Read the model definition and answer for the solid it produces. Units are mm, in the model's axes. Coordinates: 2 decimals unless noted, no trailing zeros. Order: outer loops, then holes, each group sorted by start corner. A loop starts at its lowest first (then second) coordinate and runs counter-clockwise, first axis right, second up.
Autodesk Inventor part; units mm, degrees
ref_plane "YZ Plane" through (0, 0, 0) normal (1, 0, 0) x (0, 1, 0)
ref_plane "XZ Plane" through (0, 0, 0) normal (0, 1, 0) x (-1, 0, 0)
ref_plane "XY Plane" through (0, 0, 0) normal (0, 0, 1) x (1, 0, 0)
sketch "Sketch1" plane through (0, 0, 0) normal (1, 0, 0) x (0, 1, 0)
  line L0 (-8.4509, -132.8176) -> (-8.4509, 317.1824)
  line L1 (-8.4509, 317.1824) -> (49.5047, 301.6533)
  line L2 (-8.4509, 317.1824) -> (51.5491, 317.1824) construction
  line L3 (49.5047, 301.6533) -> (49.5047, -128.3467)
  line L4 (49.5047, -128.3467) -> (-8.4509, -132.8176)
  point P0 (0, 0)
  dimension "d0" = 450
  dimension "d1" = 60
  dimension "d2" = 15
  dimension "d3" = 430
extrude "Extrusion1" add sketch "Sketch1" along normal blind 300
fillet "Fillet1" radius 5 2 edges at (150, -8.4509, 317.1824) (150, -8.4509, -132.8176)
fillet "Fillet2" radius 10 2 edges at (150, 49.5047, 301.6533) (150, 49.5047, -128.3467)
properties part number "Chassisew" material "Iron, Gray"
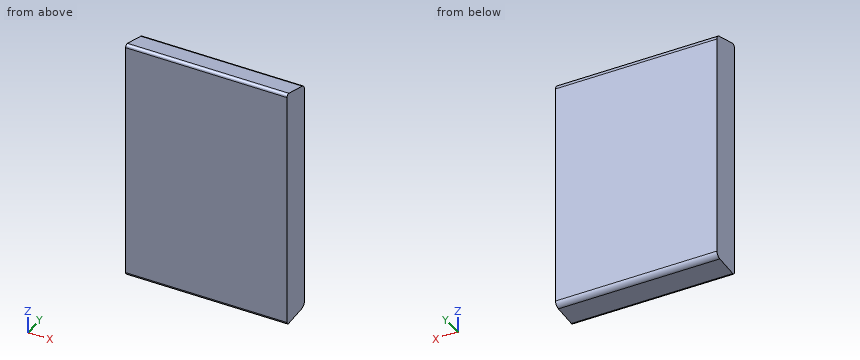
1) Straight lines are drawn through the part: line 1 (Z direction, x = 140.5, y = 21.5); line 2 (Z direction, x = 200, y = 26.5). For each, find the intervals that lie inside material, in ascending order.
A:
line 1: z = -130.51 to 309.16
line 2: z = -130.12 to 307.82
2) A cutting plane is placed at B-B, the plane y = 31. Determine the outline of the cut face in (x, z), and give its area (3 significant figures).
A:
outline: (0, -129.77) - (300, -129.77) - (300, 306.61) - (0, 306.61) - close
area: 131,000 mm2
3) Flat-ended cylindrical pins translate along their axes: pin 1 Ø12 at (y, z) = (24.5, 187) entering from -X; pin 2 Ø4 at (x, y) = (207, 30.5) entering from +Z; pin 3 Ø2 at (x, y) = (255.5, 11.5) entering from +Z; pin 4 Ø2 at (x, y) = (203.5, 3) entering from +Z. Find the tip coordinate at first contact, or state that the pin passes through.
A:
pin 1: stops at x = 0
pin 2: stops at z = 307.28
pin 3: stops at z = 312.1
pin 4: stops at z = 314.38
4) A cutting plane is placed at A-A, the plane x = 158. Determine the outline of the cut face in (y, z), and give its area (3 significant figures).
A:
outline: (-8.45, -127.42) arc R5 ccw to (-3.07, -132.4) - (40.27, -129.06) arc R10 ccw to (49.5, -119.09) - (49.5, 293.98) arc R10 ccw to (42.09, 303.64) - (-2.16, 315.5) arc R5 ccw to (-8.45, 310.67) - close
area: 25,500 mm2
